from build123d import *

# Parameters (mm, degrees)
F0_W     = 50
F0_H     = 80
F1_DEPTH = 25
F2_W     = 40
F2_H     = 33
F3_DEPTH = 25.001
F4_W     = 7
F4_H     = 25
F5_DEPTH = 3
F6_R     = 1.25
F7_DEPTH = 50.001
F8_R     = 3


with BuildPart() as f1:
    # F0 (on Front) → F1 (new body)
    with BuildSketch(Plane.XZ):
        with Locations((4.001731, 25.162706)):
            Rectangle(F0_W, F0_H)
    extrude(amount=F1_DEPTH)

    # F2 (on face) → F3 (cut, through all)
    with BuildSketch(Plane.XZ.offset(25)):
        with Locations((4.001731, 1.662706)):
            Rectangle(F2_W, F2_H)
        with Locations((4.001731, 48.662706)):
            Rectangle(F2_W, F2_H)
    extrude(amount=-F3_DEPTH, mode=Mode.SUBTRACT)

    # F4 (on face) → F5 (cut)
    with BuildSketch(Plane.YZ.offset(-15.998269)):
        with Locations((-12.5, 1.662706)):
            Rectangle(F4_W, F4_H)
        with Locations((-12.5, 48.662706)):
            Rectangle(F4_W, F4_H)
    extrude(amount=-F5_DEPTH, mode=Mode.SUBTRACT)

    # F6 (on face) → F7 (cut, through all)
    with BuildSketch(Plane(origin=(-20.998269, 0, 0), x_dir=(0, -1, 0), z_dir=(-1, 0, 0))):
        with Locations((12.5, -7.587294)):
            Circle(F6_R)
        with Locations((12.5, 57.912706)):
            Circle(F6_R)
    extrude(amount=-F7_DEPTH, mode=Mode.SUBTRACT)

    # F8
    f8_edges = [f1.edges().sort_by_distance(p)[0] for p in [
        (29.001731, -12.5, 65.162706),
        (-20.998269, -12.5, 65.162706),
        (-18.498269, 0, 65.162706),
        (26.501731, 0, 65.162706),
        (-18.498269, -25, 65.162706),
        (26.501731, -25, 65.162706),
        (29.001731, -25, 25.162706),
        (29.001731, 0, 25.162706),
        (-20.998269, -25, 25.162706),
        (-20.998269, 0, 25.162706),
        (-20.998269, -12.5, -14.837294),
        (29.001731, -12.5, -14.837294),
        (26.501731, -25, -14.837294),
        (-18.498269, -25, -14.837294),
        (26.501731, 0, -14.837294),
        (-18.498269, 0, -14.837294),
        (4.001731, -25, 18.162706),
        (4.001731, 0, 18.162706),
    ]]
    fillet(f8_edges, radius=F8_R)


solid = f1.part
For this review, take the finished solid that the model builds, in its own axes (mm). A direction names the side the tool comes from. Give positions to 0.01 mm unless a question says otherwise; leave off trailing zeros. Loops run counter-clockwise (first coordinate to the right, second up) from the corner with the lowest first, then second, coordinate; pieces in that order, holes last. Notation, with made-up numbers: M -38.75,56 L -33.75,56 A21 ccw -33.75,61 Z; hole C 53,-17.75 d2. An arc over 180 degrees is marked long. Answer as a JSON object with one key per item and string values. Group by question number.
Q1. Add section A-A on z = 39. Give the boundary of the cut face in (x, y), and give its area (3 significant figures).
Q2. Tool access review of faces 4 (the cylindrical face through (25.016, -0.855, 64.261)), 5 (the flat face through (-17, -12, 65.163)), 6 (the flat face through (-15.998, -18, 48)), 7 (the flat face through (-17, -13, 36.163)), 8 (the flat face through (4, -13, 18.163)): name each direction out of +Z, -Z, +X, -X, +Y, -Y from which nothing blocks a thin tool from reaching the whole face with its end or side.
Q3. Add section D-D on x = 6.5. Give the boundary of the cut face in (y, z), and give its area (3 significant figures).
Q4. Mouldability with a two-part tool opening along Z and no side actions: class faces 1 (the cylindrical face through (25.02, -24.14, -13.94)), 2 (the flat face through (24.002, -13, 48)), 3 (the flat face through (-17, -9, 48)) as +Z half, -Z half, draft (parallel to the pull), parting line (faces both ways), or undercut.
Q5. Insertion check: P1, Ø15, axis at x = 8.5, y = -8.5, coming from the -Z side. The pin has a flat end and moves straight along its axis. Give the tip position at first contact, or say it passes through.
Q6. Add section C-C on y = -12.5. Give the number of separate pieces and of enclosed holes in the cut face, and give its area (3 significant figures).
Q7. For probe 1 along Z at (x, y) = (27.2, -12.5); probe 2 along Z at (x, y) = (25.1, -12.5); probe 3 along X at (y, z) = (-7.5, 7), list the stretches that pass through material, from the lowest coordinate up. Write a range as [from, to].
Q8. Add section B-B on y = -20. Give the boundary of the cut face in (x, z).
Checked values:
{
 "1": {"outline": "M -21,-22 A3 ccw -18,-25 L -16,-25 L -16,-16 L -19,-16 L -19,-9 L -16,-9 L -16,0 L -18,0 A3 ccw -21,-3 Z; M 24,-25 L 26,-25 A3 ccw 29,-22 L 29,-3 A3 ccw 26,0 L 24,0 Z", "area": "221 mm²"},
 "2": {"face 4": "+Z, +X, -X, +Y", "face 5": "+Z, +X, -X, +Y, -Y", "face 6": "+Z, +Y, -Y", "face 7": "none", "face 8": "-Z, +Y, -Y"},
 "3": {"outline": "M -25,21.16 A3 ccw -22,18.16 L -3,18.16 A3 ccw 0,21.16 L 0,32.16 L -25,32.16 Z", "area": "346 mm²"},
 "4": {"face 1": "-Z half", "face 2": "draft", "face 3": "undercut"},
 "5": {"P1": "z = 18.16"},
 "6": {"separate pieces": "5", "enclosed holes": "0", "area": "1,170 mm²"},
 "7": {"probe 1": "[-14.59, -8.84], [-6.34, 56.66], [59.16, 64.91]", "probe 2": "[-14.84, -8.84], [-6.34, 56.66], [59.16, 65.16]", "probe 3": "[-21, -16], [24, 29]"},
 "8": {"outline": "M -21,-11.84 A3 ccw -18,-14.84 L -16,-14.84 L -16,18.16 L 24,18.16 L 24,-14.84 L 26,-14.84 A3 ccw 29,-11.84 L 29,62.16 A3 ccw 26,65.16 L 24,65.16 L 24,32.16 L -16,32.16 L -16,65.16 L -18,65.16 A3 ccw -21,62.16 Z"}
}
